from build123d import *

# Parameters (mm, degrees)
SKETCH1_W           = 92
SKETCH1_H           = 68
BOSS_EXTRUDE1_DEPTH = 9.5
FILLET1_R           = 3
SHELL1_T            = -2
SKETCH3_W           = 5
SKETCH3_H           = 2
BOSS_EXTRUDE2_DEPTH = 12.5
BOSS_EXTRUDE3_DEPTH = 5
CUT_EXTRUDE1_REACH  = 94
SKETCH5_W           = 12
SKETCH5_H           = 7.5
FILLET2_R           = 2


with BuildPart() as part:
    # Sketch1 → Boss-Extrude1 (new body)
    with BuildSketch(Plane(origin=(0, 0, 0), x_dir=(1, 0, 0), z_dir=(0, 1, 0))):
        Rectangle(SKETCH1_W, SKETCH1_H)
    extrude(amount=BOSS_EXTRUDE1_DEPTH)

    # Fillet1
    fillet1_edges = [part.edges().sort_by_distance(p)[0] for p in [
        (46, 4.75, 34),
        (-46, 4.75, 34),
        (-46, 4.75, -34),
        (46, 4.75, -34),
    ]]
    fillet(fillet1_edges, radius=FILLET1_R)

    # Shell1
    shell1_openings = [part.faces().sort_by_distance(p)[0] for p in [
        (0, 9.5, 0),
    ]]
    offset(amount=SHELL1_T, openings=shell1_openings, kind=Kind.INTERSECTION)

    # Sketch3 → Boss-Extrude2 (add)
    with BuildSketch(Plane(origin=(0, 2, 0), x_dir=(1, 0, 0), z_dir=(0, 1, 0))):
        with Locations((0, 31)):
            Rectangle(SKETCH3_W, SKETCH3_H)
    boss_extrude2 = extrude(amount=BOSS_EXTRUDE2_DEPTH)

    # Sketch4 → Boss-Extrude3 (add)
    with BuildSketch(Plane.ZY.offset(2.5)):
        Polygon((-32, 14.5), (-33.5, 12.712369611), (-33.5, 11.5), (-32, 11.5), align=None)
    boss_extrude3 = extrude(amount=-BOSS_EXTRUDE3_DEPTH)

    # Mirror1: Boss-Extrude2, Boss-Extrude3 across plane
    add(boss_extrude2.mirror(Plane.XY))
    add(boss_extrude3.mirror(Plane.XY))

    # Sketch5 → Cut-Extrude1 (cut, up to next)
    with BuildSketch(Plane(origin=(46, 0, 0), x_dir=(0, 0, -1), z_dir=(1, 0, 0)), mode=Mode.PRIVATE) as cut_extrude1_sk1:
        with Locations((0, 5.75)):
            Rectangle(SKETCH5_W, SKETCH5_H)
    cut_extrude1_tool1 = extrude(cut_extrude1_sk1.sketch, amount=-CUT_EXTRUDE1_REACH, mode=Mode.PRIVATE) & part.part
    add(cut_extrude1_tool1.solids().sort_by_distance((46, 5.75, 0))[0], mode=Mode.SUBTRACT)

    # Fillet2
    fillet2_edges = [part.edges().sort_by_distance(p)[0] for p in [
        (45, 2, 6),
        (45, 2, -6),
    ]]
    fillet(fillet2_edges, radius=FILLET2_R)


solid = part.part
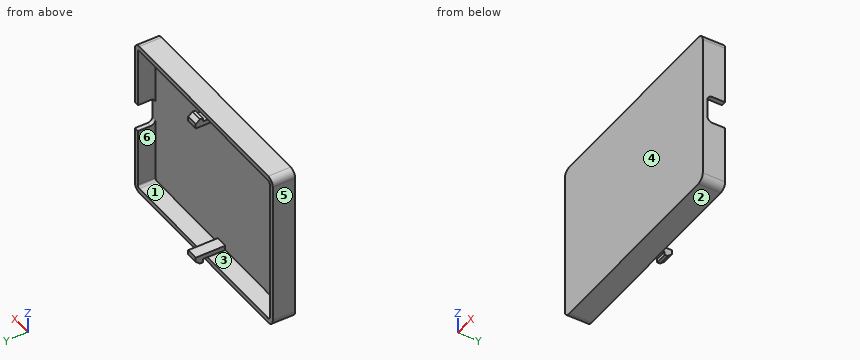
Can you work these out from the model? Positions are in its coordinate system, mm. Face numbers are marked on the shaded views. A direction names the side the tool comes from. Coordinates: 2 decimals unless noted, no trailing zeros. Order: outer loops, then holes, each group sorted by start corner. A loop starts at its lowest first (then second) coordinate and runs counter-clockwise, first axis right, second up. Notation, with made-up numbers: (-24, 41) -> (-13, 41) arc R3 ccw to (-13, 46) -> close; hole circle Ø5 at (3.25, 82.5). An arc over 180 degrees is marked (long way). Use one line per item in the form item = value.
Q1. Imagine slicing it at B-B, the plane y = 6.25. List the corners of the cut face in (x, z) for me.
From the geometry:
outline = (-46, -31) arc R3 ccw to (-43, -34) -> (43, -34) arc R3 ccw to (46, -31) -> (46, -6) -> (44, -6) -> (44, -31) arc R1 cw to (43, -32) -> (2.5, -32) -> (2.5, -30) -> (-2.5, -30) -> (-2.5, -32) -> (-43, -32) arc R1 cw to (-44, -31) -> (-44, 31) arc R1 cw to (-43, 32) -> (-2.5, 32) -> (-2.5, 30) -> (2.5, 30) -> (2.5, 32) -> (43, 32) arc R1 cw to (44, 31) -> (44, 6) -> (46, 6) -> (46, 31) arc R3 ccw to (43, 34) -> (-43, 34) arc R3 ccw to (-46, 31) -> close
Q2. Will these pins go through, and if not, where does the flat tip stop? P1, Ø0.6, axis at x = 0.5, y = 10.5, coming from the +Z side; P2, Ø1, axis at x = 1, y = 12, coming from the +Z side; P3, Ø1, axis at x = -0.5, y = 10.5, coming from the -Z side.
From the geometry:
P1 = 32
P2 = 33.5
P3 = -32
Q3. Imagine slicing it at C-C, the plane z = -16. List the corners of the cut face in (x, y) for me, then the cut area to 3 significant figures.
From the geometry:
outline = (-46, 0) -> (46, 0) -> (46, 9.5) -> (44, 9.5) -> (44, 2) -> (-44, 2) -> (-44, 9.5) -> (-46, 9.5) -> close
area = 214 mm²
Q4. I need wall thicknesses on L1, parallel to Z at x = -32.5, y = 4.25; L2, parallel to X at y = 6.25, z = 29; L3, parallel to Y at x = -38, z = -30.5. Which ranges of each line are inside material? Lowest first, please.
From the geometry:
L1 = -34 to -32, 32 to 34
L2 = -46 to -44, 44 to 46
L3 = 0 to 2
Q5. Imagine slicing it at A-A, the plane x = -39. List the corners of the cut face in (y, z) for me, then the cut area to 3 significant figures.
From the geometry:
outline = (0, -34) -> (9.5, -34) -> (9.5, -32) -> (2, -32) -> (2, 32) -> (9.5, 32) -> (9.5, 34) -> (0, 34) -> close
area = 166 mm²
Q6. We'd pull the mould along Z, two halves only. Please class the marked faces 1, 2, 3 and 4: released by +Z, released by -Z, zero draft, split by the parting line, or undercut.
From the geometry:
face_1 = undercut
face_2 = released by -Z
face_3 = undercut
face_4 = zero draft
Q7. Imagine slicing it at D-D, the plane z = -1.5. List the corners of the cut face in (x, y) for me, then the cut area to 3 significant figures.
From the geometry:
outline = (-46, 0) -> (46, 0) -> (46, 2) -> (-44, 2) -> (-44, 9.5) -> (-46, 9.5) -> close
area = 199 mm²
Q8. Which directions (+Z, -Z, +X, -X, +Y, -Y) give clear straight access to the entire face, cutting with the end or side of a thin tool? Please do the marked faces 5 and 6.
From the geometry:
face_5 = +Z, -Z, -X, +Y, -Y
face_6 = +Y
